Design review of the part built by this model. Coordinates are the model's own, in mm. Face numbers are marked on the shaded views. A direction names the side the tool comes from. Give positions to 0.01 mm unless a question says otherwise; leave off trailing zeros. Loops run counter-clockwise (first coordinate to the right, second up) from the corner with the lowest first, then second, coordinate; pieces in that order, holes last. Notation, with made-up numbers: M -9,50.25 L 17,50.25 A14 ccw 17,70.25 Z; hole C 62,84.25 d6. An arc over 180 degrees is marked long. Use a Markdown table: item, result. Add a question column.
(1) Add section B-B, the plane z = -3.5. Give the boundary of the cut face in (x, y) (3 decimals).
(2) Add section C-C, the plane y = 0. Give the boundary of the cut face in (x, z) (3 decimals), then the cut area to 3 significant figures.
(3) Draft analysis for pull direction Y (two halves, no side actions). For the marked faces 1, 2 and 3, state which applies: pulls with the +Y half, pulls with the -Y half, needs draft (parallel to the pull), parting line crosses it, or undercut.
(4) For probe 1 along Y at (x, z) = (0, -0.5) (3 decimals); probe 2 along Z at (x, y) = (3.5, -1); probe 3 along Y at (x, z) = (1.5, 5.5) (3 decimals), list the stretches that pass through material, from the lowest coordinate up.
(5) Add section A-A, the plane x = 0. Give the boundary of the cut face in (y, z) (3 decimals).
(6) Add section D-D, the plane z = 2.75. Give the boundary of the cut face in (x, y).
(7) For the marked faces 4 and 5, list the 3-axis set-ups (+Z, -Z, +X, -X, +Y, -Y) from which the entire face can be reached by the end or side of a thin tool; tool diameter is ignored.
(8) Insertion check: pin 1 Ø5 at (x, y) = (0.5, 4.5) entering from -Z; pin 2 Ø0.7 at (x, z) = (1, -2.5) entering from +Y; pin 3 Ø1.5 at (y, z) = (1, -3.5) entering from -X; pin 4 Ø0.6 at (y, z) = (1.5, 5.5) entering from +X. Each pin has a flat end and moves straight along its axis. Give the tip position at first contact, or say it passes through.
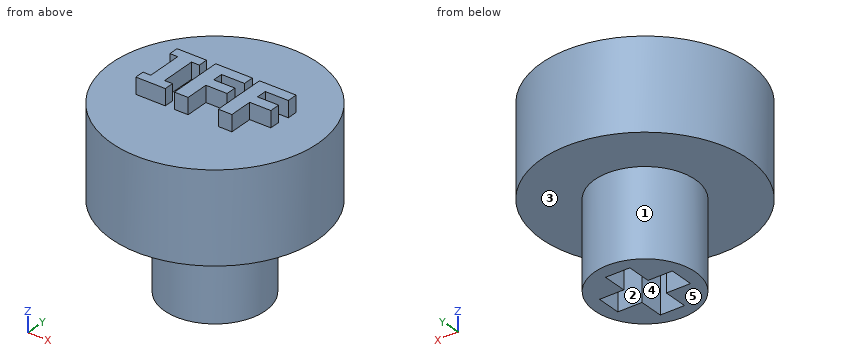
Autodesk Inventor part; units mm, degrees
ref_plane "YZ Plane" through (0, 0, 0) normal (1, 0, 0) x (0, 1, 0)
ref_plane "XZ Plane" through (0, 0, 0) normal (0, 1, 0) x (-1, 0, 0)
ref_plane "XY Plane" through (0, 0, 0) normal (0, 0, 1) x (1, 0, 0)
sketch "Sketch1" plane through (0, 0, 0) normal (0, 0, 1) x (1, 0, 0)
  circle A0 centre (0, 0) radius 6.22 construction
  circle A1 centre (0, 0) radius 2.8
  line L0 (-0.675, 0.675) -> (-0.675, 2.025)
  line L1 (-0.675, 2.025) -> (0.675, 2.025)
  line L2 (0.675, 2.025) -> (0.675, 0.675)
  line L3 (0.675, 0.675) -> (2.025, 0.675)
  line L4 (2.025, 0.675) -> (2.025, -0.675)
  line L5 (2.025, -0.675) -> (0.675, -0.675)
  line L6 (0.675, -0.675) -> (0.675, -2.025)
  line L7 (0.675, -2.025) -> (-0.675, -2.025)
  line L8 (-0.675, -2.025) -> (-0.675, -0.675)
  line L9 (-0.675, -0.675) -> (-2.025, -0.675)
  line L10 (-2.025, -0.675) -> (-2.025, 0.675)
  line L11 (-2.025, 0.675) -> (-0.675, 0.675)
  circle A2 centre (0, 0) radius 5.75
  point P0 (-6.07, -6.1)
  dimension "d0" = 12.44
  dimension "d1" = 0.47
extrude "Extrusion1" add sketch "Sketch1" along normal blind 5 contours A1 | L0 L1 L2 L3 L4 L5 L6 L7 L8 L9 L10 L11 | A2
extrude "Extrusion2" add sketch "Sketch1" against normal blind 4.8 contours A1
sketch "Sketch2" plane through (0, 0, 5) normal (0, 0, 1) x (1, 0, 0)
  point P0 (0, 0)
sketch "Sketch3" plane through (0, 0, 5) normal (0, 0, 1) x (1, 0, 0)
  line L0 (-3.4504, 1.525) -> (3.4504, 1.525) construction
  line L1 (3.4504, 1.525) -> (3.4504, -1.525) construction
  line L2 (3.4504, -1.525) -> (-3.4504, -1.525) construction
  line L3 (-3.4504, -1.525) -> (-3.4504, 1.525) construction
  line L4 (-1.6165, -1.525) -> (-3.2576, -1.525)
  line L5 (-3.2576, -1.525) -> (-3.2576, -0.9936)
  line L6 (-3.2576, -0.9936) -> (-2.8201, -0.9936)
  line L7 (-2.8201, -0.9936) -> (-2.8201, 0.9936)
  line L8 (-2.8201, 0.9936) -> (-3.2576, 0.9936)
  line L9 (-3.2576, 0.9936) -> (-3.2576, 1.525)
  line L10 (-3.2576, 1.525) -> (-1.6165, 1.525)
  line L11 (-1.6165, 1.525) -> (-1.6165, 0.9936)
  line L12 (-1.6165, 0.9936) -> (-2.0539, 0.9936)
  line L13 (-2.0539, 0.9936) -> (-2.0539, -0.9936)
  line L14 (-2.0539, -0.9936) -> (-1.6165, -0.9936)
  line L15 (-1.6165, -0.9936) -> (-1.6165, -1.525)
  line L16 (0.9343, 0.9442) -> (-0.346, 0.9442)
  line L17 (-0.346, 0.9442) -> (-0.346, 0.3683)
  line L18 (-0.346, 0.3683) -> (0.8329, 0.3683)
  line L19 (0.8329, 0.3683) -> (0.8329, -0.2126)
  line L20 (0.8329, -0.2126) -> (-0.346, -0.2126)
  line L21 (-0.346, -0.2126) -> (-0.346, -1.525)
  line L22 (-0.346, -1.525) -> (-1.1073, -1.525)
  line L23 (-1.1073, -1.525) -> (-1.1073, 1.525)
  line L24 (-1.1073, 1.525) -> (0.9343, 1.525)
  line L25 (0.9343, 1.525) -> (0.9343, 0.9442)
  line L26 (3.3713, 0.9442) -> (2.091, 0.9442)
  line L27 (2.091, 0.9442) -> (2.091, 0.3683)
  line L28 (2.091, 0.3683) -> (3.27, 0.3683)
  line L29 (3.27, 0.3683) -> (3.27, -0.2126)
  line L30 (3.27, -0.2126) -> (2.091, -0.2126)
  line L31 (2.091, -0.2126) -> (2.091, -1.525)
  line L32 (2.091, -1.525) -> (1.3297, -1.525)
  line L33 (1.3297, -1.525) -> (1.3297, 1.525)
  line L34 (1.3297, 1.525) -> (3.3713, 1.525)
  line L35 (3.3713, 1.525) -> (3.3713, 0.9442)
  point P0 (0, 0)
  point P1 (0, -1.525)
  point P2 (0, 0)
extrude "Extrusion4" add sketch "Sketch3" along normal blind 0.9
properties part number "IPC IFF"
Established:
| question | item | result |
|---|---|---|
| 1 | outline | C 0,0 d5.6; hole M -2.025,-0.675 L -0.675,-0.675 L -0.675,-2.025 L 0.675,-2.025 L 0.675,-0.675 L 2.025,-0.675 L 2.025,0.675 L 0.675,0.675 L 0.675,2.025 L -0.675,2.025 L -0.675,0.675 L -2.025,0.675 Z |
| 2 | outline | M -5.75,0 L -2.8,0 L -2.8,-4.8 L -2.025,-4.8 L -2.025,0 L 2.025,0 L 2.025,-4.8 L 2.8,-4.8 L 2.8,0 L 5.75,0 L 5.75,5 L 3.27,5 L 3.27,5.9 L 1.33,5.9 L 1.33,5 L 0.833,5 L 0.833,5.9 L -1.107,5.9 L -1.107,5 L -2.054,5 L -2.054,5.9 L -2.82,5.9 L -2.82,5 L -5.75,5 Z |
| 2 | area | 69.1 mm^2 |
| 3 | face 1 | parting line crosses it |
| 3 | face 2 | undercut |
| 3 | face 3 | needs draft |
| 4 | probe 1 | -2.8 to -2.025, 2.025 to 2.8 |
| 4 | probe 2 | 0 to 5 |
| 4 | probe 3 | -1.525 to 1.525 |
| 5 | outline | M -5.75,0 L -2.8,0 L -2.8,-4.8 L -2.025,-4.8 L -2.025,0 L 2.025,0 L 2.025,-4.8 L 2.8,-4.8 L 2.8,0 L 5.75,0 L 5.75,5 L 1.525,5 L 1.525,5.9 L 0.944,5.9 L 0.944,5 L 0.368,5 L 0.368,5.9 L -0.213,5.9 L -0.213,5 L -5.75,5 Z |
| 6 | outline | C 0,0 d11.5 |
| 7 | face 4 | -Z |
| 7 | face 5 | -Z, +X, -X, +Y, -Y |
| 8 | pin 1 | z = -4.8 |
| 8 | pin 2 | y = 2.72 |
| 8 | pin 3 | x = -2.79 |
| 8 | pin 4 | x = 3.37 |
